Drawing for the job (mm, zero at the part's lowest x, y, z). A direction names the side the tool comes from. Give positions to 0.01 mm unless a question says otherwise; leave off trailing zeros. Order: outer loops, then holes, each group sorted by start corner. A loop starts at its lowest first (then second) coordinate and runs counter-clockwise, first axis right, second up. Notation, with made-up numbers: (73, 3) -> (83, 3) arc R27 ccw to (83, 26) -> close; hole circle Ø6 at (-24.5, 37). An arc over 180 degrees is marked (long way). One line per item, written item: value. Start each with the question number.
(1) Saw through at C-C on y = 21.45. Give the cut face in (x, z).
(2) Saw through at A-A on z = 3.9. Give the cut face in (x, y), plus the area to 3 significant figures.
(3) Pin check, flat tips, straight feed: pin 1 (1 mm diameter, centred on y = 41, z = 4, fed in from -X); pin 2 (1 mm diameter, centred on x = 15, y = 18, fed in from +Z); pin 3 (2.5 mm diameter, centred on x = 41.5, z = 3, fed in from -Y); pin 4 (1.5 mm diameter, centred on x = 12.5, y = 30.5, fed in from -Z). Stop position of each tip, or through.
(4) Probe line 1 (Z direction, x = 2.5, y = 23.5); line 2 (X direction, y = 21, z = 4.25) (1 decimal); line 3 (Y direction, x = 20, z = 3.4). List the from-to ranges inside material, lowest first.
(5) Which spindle directions (+Z, -Z, +X, -X, +Y, -Y) get a long thin tool onto all of the face, cutting with end or side? Do the marked faces 1, 2 and 3. Say none if no direction does.
(6) Saw through at B-B on x = 21.45. Give the cut face in (y, z).
(7) Saw through at D-D on y = 37.5. Give the cut face in (x, z).
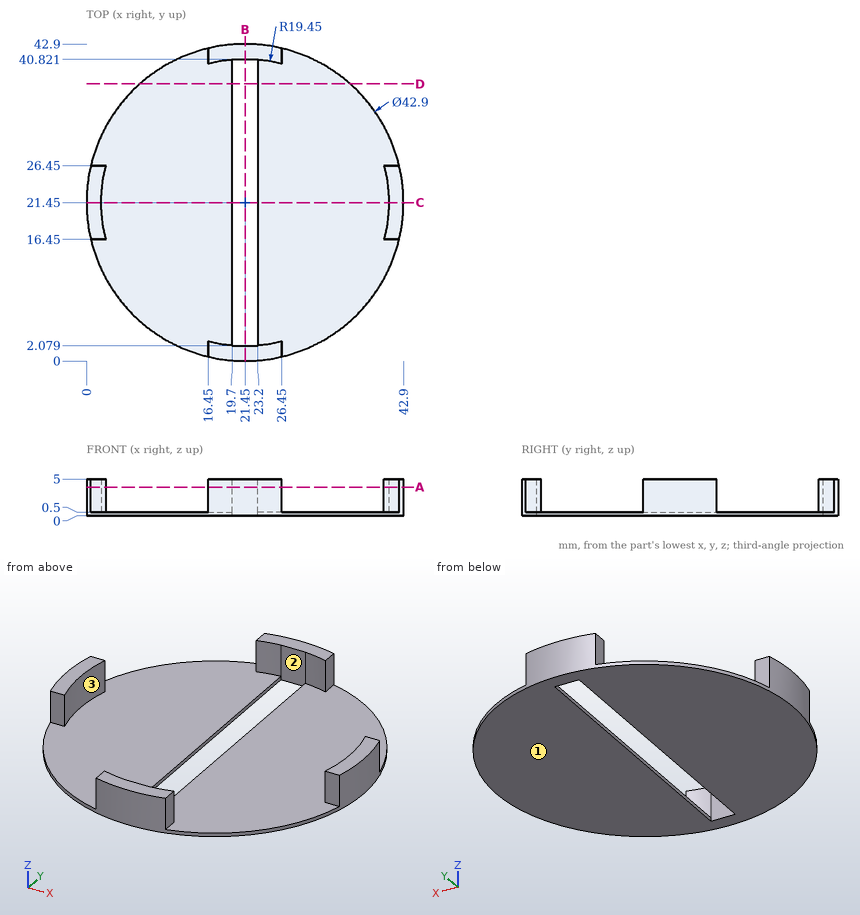
Results below:
1. outline: (0, 0) -> (19.7, 0) -> (19.7, 0.5) -> (2, 0.5) -> (2, 5) -> (0, 5) -> close; (23.2, 0) -> (42.9, 0) -> (42.9, 5) -> (40.9, 5) -> (40.9, 0.5) -> (23.2, 0.5) -> close
2. outline: (0.59, 16.45) -> (2.65, 16.45) arc R19.45 cw to (2.65, 26.45) -> (0.59, 26.45) arc R21.45 ccw to start; (16.45, 0.59) arc R21.45 ccw to (26.45, 0.59) -> (26.45, 2.65) arc R19.45 cw to (23.2, 2.08) -> (19.7, 2.08) arc R19.45 cw to (16.45, 2.65) -> close; (16.45, 40.25) arc R19.45 cw to (19.7, 40.82) -> (23.2, 40.82) arc R19.45 cw to (26.45, 40.25) -> (26.45, 42.31) arc R21.45 ccw to (16.45, 42.31) -> close; (40.25, 16.45) -> (42.31, 16.45) arc R21.45 ccw to (42.31, 26.45) -> (40.25, 26.45) arc R19.45 cw to start
2. area: 81.2 mm²
3. pin 1: stops at x = 16.45
3. pin 2: stops at z = 0.5
3. pin 3: stops at y = 16.45
3. pin 4: stops at z = 0
4. line 1: z = 0 to 0.5
4. line 2: x = 0 to 2, 40.9 to 42.9
4. line 3: y = 0.05 to 2.08, 40.82 to 42.85
5. face 1: -Z, +X, -X, +Y, -Y
5. face 2: +Z, -Z
5. face 3: +Z
6. outline: (0, 0) -> (2.08, 0) -> (2.08, 5) -> (0, 5) -> close; (40.82, 0) -> (42.9, 0) -> (42.9, 5) -> (40.82, 5) -> close
7. outline: (7.22, 0) -> (19.7, 0) -> (19.7, 0.5) -> (7.22, 0.5) -> close; (23.2, 0) -> (35.68, 0) -> (35.68, 0.5) -> (23.2, 0.5) -> close
